Autodesk Inventor part; units mm, degrees
ref_plane "YZ Plane" through (0, 0, 0) normal (1, 0, 0) x (0, 1, 0)
ref_plane "XZ Plane" through (0, 0, 0) normal (0, 1, 0) x (-1, 0, 0)
ref_plane "XY Plane" through (0, 0, 0) normal (0, 0, 1) x (1, 0, 0)
sketch "Sketch1" plane through (0, 0, 0) normal (0, 0, 1) x (1, 0, 0)
  line L0 (0, 0) -> (3.81, 0)
  line L1 (0, 0) -> (0, 1.27)
  arc A0 (3.81, 0) -> (1.359061, 1.27) centre (3.81, 3) ccw
  circle A1 centre (3.81, 3) radius 1.9
  line L2 (0, 1.27) -> (1.359061, 1.27)
  dimension "d0" = 3.81
  dimension "d1" = 1.27
  dimension "d2" = 6
  dimension "d3" = 3.8
extrude "Extrusion1" add sketch "Sketch1" along normal blind 30.48
ref_plane "Work Plane1" through (0, 0, 20.32) normal (0, 0, 1) x (1, 0, 0)
sketch "Sketch2" plane through (0, 0, 20.32) normal (0, 0, 1) x (1, 0, 0)
  arc A0 (3.81, 0) -> (1.359061, 1.27) centre (3.81, 3) ccw
  line L0 (2.54, 1.27) -> (2.54, 0)
  line L1 (0, 0) -> (3.81, 0)
  line L2 (2.54, 0) -> (3.81, 0)
  circle A1 centre (3.81, 3) radius 0.762
sketch "Sketch2 outline for Extrusion2" plane through (0, 0, 20.32) normal (0, 0, 1) x (1, 0, 0)
  line L0 (2.54, 0) -> (3.81, 0)
  line L1 (1.359061, 1.27) -> (2.54, 0)
  arc A0 (3.81, 0) -> (1.359061, 1.27) centre (3.81, 3) ccw
  circle A1 centre (3.81, 3) radius 0.762
extrude "Extrusion2" cut sketch "Sketch2 outline for Extrusion2" against normal blind 10.16
sketch "Sketch3" plane through (0, 1.27, 0) normal (0, 1, 0) x (1, 0, 0)
  line L0 (0, 0) -> (3.81, 0)
  line L1 (0, 0) -> (2.531995, 0)
  line L2 (2.531995, 0) -> (-25.408005, 0)
  line L3 (-25.408005, 0) -> (-25.408005, -27.94)
  line L4 (-25.408005, -27.94) -> (2.531995, -27.94)
  line L5 (1.359061, 0) -> (1.359061, -10.16)
  line L6 (1.359061, 0) -> (1.359061, -1.27)
  line L7 (1.359061, -1.27) -> (-25.310939, -1.27)
  line L8 (1.359061, -20.32) -> (1.359061, -30.48)
  line L9 (1.359061, -30.48) -> (1.359061, -29.21)
  line L10 (1.359061, -29.21) -> (-25.310939, -29.21)
  line L11 (-25.310939, -29.21) -> (-25.310939, -1.27)
  line L12 (0.085059, -1.27) -> (0.085059, -29.21)
  line L13 (0, 0) -> (0, -30.48)
  line L14 (0, -1.27) -> (0, -29.21)
  line L15 (1.359061, -29.21) -> (1.359061, -30.48)
  line L16 (1.359061, 0) -> (1.359061, -1.27)
  line L17 (1.359061, -30.48) -> (1.359061, -29.21)
  line L18 (1.359061, -30.48) -> (6.81, -30.48)
  line L19 (1.359061, -30.48) -> (-1.399798, -27.94)
  line L20 (1.359061, -30.48) -> (1.359061, -29.21)
  line L21 (1.359061, -29.21) -> (-1.466488, -29.21)
  point P0 (3.81, -30.48)
  dimension "d9" = 27.94
  dimension "d10" = 27.94
  dimension "d11" = 27.94
  dimension "d12" = 1.27
  dimension "d13" = 26.67
  dimension "d14" = 1.27
  dimension "d15" = 26.67
extrude "Extrusion3" cut sketch "Sketch3" against normal blind 25.4 contours L7 L12 L4 L13 | L4 L12 L10 L13
sketch "Sketch4" plane through (0, 0, 0) normal (0, -1, 0) x (1, 0, 0)
  line L0 (1.359061, 0) -> (1.359061, 10.16)
  line L1 (1.359061, 0) -> (-29.120939, 0)
  line L2 (-29.120939, 0) -> (-29.120939, 30.48)
  line L3 (-29.120939, 30.48) -> (1.359061, 30.48)
  line L4 (1.359061, 30.48) -> (1.359061, 0)
  line L5 (0, 1.27) -> (0.085059, 1.27)
  line L6 (0.085059, 1.27) -> (-27.854941, 1.27)
  line L7 (-27.854941, 1.27) -> (-27.854941, 29.21)
  line L8 (-27.854941, 29.21) -> (0.085059, 29.21)
  line L9 (0.085059, 29.21) -> (0.085059, 1.27)
  point P0 (0, 0)
  dimension "d18" = 30.48
  dimension "d19" = 30.48
  dimension "d20" = 30.48
  dimension "d21" = 27.94
  dimension "d22" = 27.94
  dimension "d23" = 27.94
sketch "Sketch5" plane through (0, 1.27, 0) normal (0, 1, 0) x (1, 0, 0)
  line L0 (1.359061, 0) -> (0, 0)
  line L1 (1.359061, 0) -> (0, 0)
  line L2 (0, 0) -> (0, -1.27)
  line L3 (0, 0) -> (0, -1.27)
  line L4 (0, -1.27) -> (1.359061, -1.27)
  line L5 (1.359061, 0) -> (1.359061, -10.16)
  line L6 (0, -29.21) -> (0, -30.48)
  line L7 (0, -29.21) -> (2.54, -29.21)
  line L8 (2.54, -29.21) -> (2.54, -30.48)
  line L9 (2.54, -30.48) -> (0, -30.48)
  line L10 (0, -30.48) -> (0, -29.21)
extrude "Extrusion4" cut sketch "Sketch5" against normal blind 25.4
sketch "Sketch6" plane through (1.359061, 1.27, 20.32) normal (0, 1, 0) x (1, 0, 0)
  line L0 (0, 19.05) -> (0, 10.16)
  line L1 (0, 0) -> (0, 10.16)
  line L2 (0, 19.05) -> (0, -8.89)
  line L3 (-1.274003, -8.89) -> (-1.274003, 19.05)
  line L4 (0, -8.89) -> (-1.274003, -8.89)
  line L5 (-1.274003, -8.89) -> (-1.274003, 19.05)
  line L6 (-1.274003, 19.05) -> (0, 19.05)
  point P0 (-1.359061, 20.32)
extrude "Extrusion5" cut sketch "Sketch6" against normal blind 25.4
extrude "Extrusion6" add sketch "Sketch4" against normal blind 1.27
sketch "Sketch7" plane through (0, 1.27, 0) normal (0, 1, 0) x (1, 0, 0)
  line L0 (1.359061, -29.21) -> (1.359061, -30.48)
  line L1 (-29.120939, 0) -> (-29.120939, -30.48)
  line L2 (2.54, 0) -> (-29.120939, 0)
  line L3 (-29.120939, 0) -> (-29.120939, -30.48)
  line L4 (-29.120939, -30.48) -> (2.54, -30.48)
  line L5 (2.54, -30.48) -> (2.54, 0)
  point P0 (0, 0)
  point P1 (2.54, -9.31335)
extrude "Extrusion7" add sketch "Sketch7" along normal blind 1.27
sketch "Sketch8" plane through (0, 2.54, 0) normal (0, 1, 0) x (1, 0, 0)
  line L0 (-22.120939, 7.26) -> (-22.120939, -37.74)
  line L1 (-29.120939, 0) -> (-29.120939, -30.48)
  line L2 (-29.120939, 0) -> (-29.120939, -30.48)
  line L3 (-29.120939, 0) -> (-26.370939, 0)
  line L4 (-26.370939, 0) -> (-26.370939, -30.48)
  line L5 (-26.370939, -30.48) -> (-29.120939, -30.48)
  line L6 (-29.120939, -30.48) -> (-29.120939, 0)
  point P0 (0, 0)
  dimension "d32" = 2.75
extrude "Extrusion8" add sketch "Sketch8" along normal blind 22
sketch "Sketch9" plane through (0, 0, 0) normal (0, 0, -1) x (-1, 0, 0)
  arc A0 (-0.845476, 2.54) -> (-3.81, 0) centre (-3.81, 3) ccw
  line L0 (29.120939, 0) -> (-3.81, 0)
  line L1 (29.120939, 0) -> (29.120939, 24.54)
  line L2 (26.370939, 24.54) -> (29.120939, 24.54)
  line L3 (26.370939, 2.54) -> (26.370939, 24.54)
  line L4 (-0.845476, 2.54) -> (26.370939, 2.54)
  line L5 (-2.54, 1.586812) -> (-2.54, 2.54)
  arc A1 (-1.966525, 2.54) -> (-2.54, 1.586812) centre (-3.81, 3) ccw
  line L6 (-2.54, 2.54) -> (-1.966525, 2.54)
  point P0 (0, 0)
extrude "Extrusion9" add sketch "Sketch9" along normal blind 10
sketch "Sketch10" plane through (0, 0, 30.48) normal (0, 0, 1) x (1, 0, 0)
  line L0 (0.085059, 1.27) -> (-27.854941, 1.27)
  line L1 (-26.370939, 2.54) -> (2.54, 2.54)
  line L2 (2.54, 0) -> (3.81, 0)
  arc A0 (3.81, 0) -> (0.845476, 2.54) centre (3.81, 3) ccw
  line L3 (2.54, 1.586812) -> (2.54, 2.54)
  line L4 (1.966525, 2.54) -> (2.54, 2.54)
  line L5 (-26.370939, 2.54) -> (-26.370939, 24.54)
  line L6 (-29.120939, 24.54) -> (-26.370939, 24.54)
  line L7 (-29.120939, 0) -> (-29.120939, 24.54)
  arc A1 (2.54, 1.586812) -> (1.966525, 2.54) centre (3.81, 3) ccw
  line L8 (1.359061, 1.27) -> (2.54, 1.27)
  line L9 (2.54, 1.27) -> (2.54, 0)
  line L10 (-26.370939, 2.54) -> (0.845476, 2.54)
  line L11 (-29.120939, 0) -> (1.359061, 0)
  line L12 (1.359061, 0) -> (1.359061, 1.27)
  point P0 (0, 0)
extrude "Extrusion10" add sketch "Sketch10" along normal blind 10
fillet "Fillet1" radius 3.175 2 edges at (-27.7459, 24.54, -10) (-27.7459, 24.54, 40.48)
sketch "Sketch12" plane through (0, 0, 40.48) normal (0, 0, 1) x (1, 0, 0)
  line L0 (2.54, 1.27) -> (2.54, 0)
  line L1 (1.359061, 1.27) -> (2.54, 1.27)
  line L2 (1.359061, 1.27) -> (1.359061, 0)
  line L3 (2.54, 0) -> (1.359061, 0)
  line L4 (2.54, 1.27) -> (2.54, 0)
  line L5 (2.54, 1.27) -> (1.359061, 1.27)
  point P0 (0, 0)
extrude "Extrusion12" add sketch "Sketch12" against normal blind 12
sketch "Sketch13" plane through (0, 0, 40.48) normal (0, 0, 1) x (1, 0, 0)
  arc A0 (2.54, 1.586812) -> (1.966525, 2.54) centre (3.81, 3) ccw
  circle A1 centre (3.81, 3) radius 2
  point P0 (0, 0)
extrude "Extrusion13" cut sketch "Sketch13" against normal blind 5054.6
sketch "Sketch14" plane through (0, 0, 20.32) normal (0, 0, -1) x (-1, 0, 0)
  arc A0 (-1.863619, 2.54) -> (-2.54, 1.454976) centre (-3.81, 3) ccw
  line L0 (-1.863619, 2.54) -> (-0.845476, 2.54)
  arc A1 (-0.845476, 2.54) -> (-3.81, 0) centre (-3.81, 3) ccw
  line L1 (-2.54, 0) -> (-3.81, 0)
  line L2 (-1.359061, 1.27) -> (-2.54, 0)
  line L3 (-1.359061, 1.27) -> (-2.54, 1.27)
  line L4 (-2.54, 1.27) -> (-2.54, 1.454976)
  line L5 (-2.54, 1.27) -> (-2.54, 0)
  line L6 (-2.54, 1.27) -> (-1.359061, 1.27)
  line L7 (-0.845476, 2.54) -> (26.370939, 2.54)
  line L8 (-1.359061, 1.27) -> (-2.54, 0)
  point P0 (0, 0)
extrude "Extrusion14" add sketch "Sketch14" along normal blind 15 contours L3 L2 L5
sketch "Sketch15" plane through (0, 2.54, 0) normal (0, 1, 0) x (1, 0, 0)
  line L0 (0.845476, 10) -> (0.845476, -10.16)
  line L1 (1.81, -40.48) -> (1.81, 10)
  line L2 (0.845476, -10.16) -> (1.81, -10.16)
  line L3 (1.81, -10.16) -> (1.81, -20.32)
  line L4 (1.81, -20.32) -> (0.845476, -20.32)
  line L5 (0.845476, -20.32) -> (0.845476, -10.16)
  line L6 (0.845476, -10.16) -> (12.384081, -10.16)
  line L7 (12.384081, -10.16) -> (12.384081, -20.32)
  line L8 (12.384081, -20.32) -> (0.845476, -20.32)
  line L9 (0.845476, -20.32) -> (0.845476, -10.16)
  point P0 (0, 0)
extrude "Extrusion15" cut sketch "Sketch15" against normal blind 15
sketch "Sketch16" plane through (-29.120939, 0, -10) normal (-1, 0, 0) x (0, 0, 1)
  circle A0 centre (12.24, 12.54) radius 8
  circle A1 centre (38.24, 12.54) radius 8
  circle A2 centre (12.24, 12.54) radius 8.5
  circle A3 centre (38.24, 12.54) radius 8.5
  point P0 (10, 0)
  dimension "d54" = 17
  dimension "d55" = 17
extrude "Extrusion16" cut sketch "Sketch16" against normal blind 25.4 contours A0 | A1 | A2 | A3
sketch "Sketch17" plane through (0, 0, 10.16) normal (0, 0, 1) x (1, 0, 0)
  line L0 (3.81, 0) -> (0.845476, 0)
  arc A0 (3.81, 0) -> (0.845476, 2.54) centre (3.81, 3) ccw
  line L1 (0.845476, 2.54) -> (0.845476, 0)
  circle A1 centre (3.81, 3) radius 2
  point P0 (0, 0)
extrude "Extrusion17" cut sketch "Sketch17" against normal blind 0.5
sketch "Sketch18" plane through (0, 0, 20.32) normal (0, 0, -1) x (-1, 0, 0)
  circle A0 centre (-3.81, 3) radius 2
  line L0 (-0.845476, 0) -> (-3.81, 0)
  line L1 (-0.845476, 2.54) -> (-0.845476, 0)
  arc A1 (-0.845476, 2.54) -> (-3.81, 0) centre (-3.81, 3) ccw
  point P0 (0, 0)
extrude "Extrusion18" cut sketch "Sketch18" against normal blind 0.5
sketch "Sketch19" plane through (-29.120939, 0, -10) normal (0, -1, 0) x (1, 0, 0)
  line L0 (29.205997, 11.27) -> (1.265997, 11.27)
  line L1 (1.265997, 11.27) -> (1.265997, 39.21)
  line L2 (1.265997, 39.21) -> (29.205997, 39.21)
  line L3 (29.205997, 39.21) -> (29.205997, 11.27)
  point P0 (29.120939, 10)
extrude "Extrusion19" add sketch "Sketch19" against normal blind 2.032
sketch "Sketch20" plane through (-29.120939, 0, -10) normal (-1, 0, 0) x (0, 0, 1)
  line L0 (0, 2.54) -> (50.48, 2.54)
  line L1 (25.24, 2.54) -> (30.828, 2.54)
  line L2 (30.828, 2.54) -> (19.652, 2.54)
  line L3 (19.652, 2.54) -> (30.828, 2.54)
  line L4 (30.828, 2.54) -> (30.828, 5.08)
  line L5 (30.828, 5.08) -> (19.652, 5.08)
  line L6 (19.652, 5.08) -> (19.652, 2.54)
  point P0 (10, 0)
  dimension "d64" = 5.588
  dimension "d65" = 11.176
  dimension "d66" = 2.54
extrude "Extrusion20" cut sketch "Sketch20" against normal blind 25.4
fillet "Fillet2" radius 0.25 4 edges at (-27.7459, 5.08, 9.652) (-27.7459, 2.54, 9.652) (-27.7459, 2.54, 20.828) (-27.7459, 5.08, 20.828)
sketch "Sketch21" plane through (0, 2.54, 0) normal (0, 1, 0) x (1, 0, 0)
  line L0 (0.845476, -9.66) -> (0.845476, -20.82)
  line L1 (0.845476, -15.24) -> (-4.154524, -15.24)
  line L2 (-4.154524, -15.24) -> (-9.154524, -15.24)
  circle A0 centre (-9.154524, -15.24) radius 1.5
  point P0 (0, 0)
  dimension "d70" = 5
  dimension "d71" = 5
  dimension "d72" = 3
extrude "Extrusion21" cut sketch "Sketch21" against normal blind 25.4
properties part number "Lid, Explosion Button"
Input: part model. Units: mm. Frame: model coordinates. A direction names the side the tool comes from. Round coordinates to 2 decimals unless told otherwise and drop trailing zeros. Order: outer loops, then holes, each group sorted by start corner. A loop starts at its lowest first (then second) coordinate and runs counter-clockwise, first axis right, second up. Notation, with made-up numbers: (26.25, 83.25) - (43.25, 83.25) arc R20 cw to (43.25, 88.25) - close; hole circle Ø3 at (-37, 43). An arc over 180 degrees is marked (long way). Answer as a JSON object with one key per item and string values. Group by question number.
(1) Material intervals for probe 1 along X at (y, z) = (1.2, 15.24); probe 2 along Z at (x, y) = (-27, 4); probe 3 along X at (y, z) = (19.75, 17), sorted ascending. Write a range as from..to.
(2) Draft query along X for faces 3 (the face through (-26.371, 13, 15)), 4 (the face through (0.845, 1, 15)), 5 (the face through (-28, 24.54, 15)). Return one class per face: released by +X, released by -X, zero draft, split by the parting line, or undercut.
(3) Cut plane A-A (z = 2.24). Return loops of the section in (x, y).
(4) Pin query (flat end, axial travel): P1, Ø1.5, axis at x = -24, y = 11.5, coming from the +Z side; P2, Ø8, axis at x = -1, z = 31, coming from the +Y side; P3, Ø11, axis at y = 11, z = 4, coming from the +X side; P4, Ø1.3, axis at y = 1, z = 14.5, coming from the +X side. Return the tip coordinate at first contact, or that it passes through.
(5) Cut plane B-B (z = 17.5). Return loops of the section in (x, y), then the cut area to 3 significant figures.
(6) Reachability of faces 1 (the face through (-27.77, 12.91, 19.75)), 2 (the face through (-19, 2, 40.48)) from +Z, -Z, +X, -X, +Y, -Y: full face, straight path, thin tool, end or side. Return the list, or none.
(7) Cut plane D-D (x = -8.5). Return loops of the section in (y, z).
(8) Cut plane C-C (y = 19.5). Return loops of the section in (x, z).
Here are the results:
{
 "1": {"probe 1": "x = -29.12..-10.65, -7.65..0.85", "probe 2": "z = -10..9.65, 20.83..40.48", "probe 3": "x = -29.12..-26.37"},
 "2": {"face 3": "undercut", "face 4": "released by +X", "face 5": "zero draft"},
 "3": {"outline": "(-29.12, 0) - (3.81, 0) arc R3 ccw (long way) to (0.85, 2.54) - (-26.37, 2.54) - (-26.37, 4.04) - (-29.12, 4.04) - close; (-29.12, 21.04) - (-26.37, 21.04) - (-26.37, 24.54) - (-29.12, 24.54) - close; hole circle Ø4 at (3.81, 3)"},
 "4": {"P1": "passes through", "P2": "stops at y = 5.89", "P3": "stops at x = 5.47", "P4": "stops at x = 0.85"},
 "5": {"outline": "(-29.12, 0) - (0.85, 0) - (0.85, 2.54) - (-29.12, 2.54) - close; (-29.12, 5.08) - (-26.37, 5.08) - (-26.37, 24.54) - (-29.12, 24.54) - close", "area": "130 mm^2"},
 "6": {"face 1": "-X", "face 2": "+Z, +X, -X, +Y, -Y"},
 "7": {"outline": "(0, -10) - (2.54, -10) - (2.54, 13.89) - (0, 13.89) - close; (0, 16.59) - (2.54, 16.59) - (2.54, 40.48) - (0, 40.48) - close"},
 "8": {"outline": "(-29.12, -10) - (-26.37, -10) - (-26.37, -2.64) - (-29.12, -2.64) - close; (-29.12, 7.12) - (-26.37, 7.12) - (-26.37, 23.36) - (-29.12, 23.36) - close; (-29.12, 33.12) - (-26.37, 33.12) - (-26.37, 40.48) - (-29.12, 40.48) - close"}
}
